from build123d import *

# Parameters (mm, degrees)
F1_DEPTH = 6.35
F3_DEPTH = 19.05
F4_SIZE  = 1.27


with BuildPart() as f1:
    # F0 (on Top) → F1 (new body)
    with BuildSketch(Plane.XY):
        with BuildLine():
            Line((-31.75, -19.05), (31.75, -19.05))
            Line((31.75, -19.05), (31.75, 12.7))
            ThreePointArc((31.75, 12.7), (29.8901280605, 17.1901280605), (25.4, 19.05))
            Line((25.4, 19.05), (12.7, 19.05))
            ThreePointArc((12.7, 19.05), (0, 6.35), (-12.7, 19.05))
            Line((-12.7, 19.05), (-25.4, 19.05))
            ThreePointArc((-25.4, 19.05), (-29.8901280605, 17.1901280605), (-31.75, 12.7))
            Line((-31.75, 12.7), (-31.75, -19.05))
        make_face()
    extrude(amount=F1_DEPTH)

    # F2 (on face) → F3 (join)
    with BuildSketch(Plane.XY.offset(6.35)):
        with BuildLine():
            Line((-25.4, 0), (-25.4, -19.05))
            Line((-25.4, -19.05), (-19.05, -19.05))
            Line((-19.05, -19.05), (-19.05, -6.35))
            Line((-19.05, -6.35), (19.05, -6.35))
            Line((19.05, -6.35), (19.05, -19.05))
            Line((19.05, -19.05), (25.4, -19.05))
            Line((25.4, -19.05), (25.4, 0))
            Line((25.4, 0), (21.59, 0))
            ThreePointArc((21.59, 0), (17.0998719395, 1.8598719395), (15.24, 6.35))
            Line((15.24, 6.35), (15.24, 19.05))
            Line((15.24, 19.05), (12.7, 19.05))
            ThreePointArc((12.7, 19.05), (0, 6.35), (-12.7, 19.05))
            Line((-12.7, 19.05), (-15.24, 19.05))
            Line((-15.24, 19.05), (-15.24, 6.35))
            ThreePointArc((-15.24, 6.35), (-17.0998719395, 1.8598719395), (-21.59, 0))
            Line((-21.59, 0), (-25.4, 0))
        make_face()
    extrude(amount=F3_DEPTH)

    # F4
    f4_edges = [f1.edges().sort_by_distance(p)[0] for p in [
        (0, 6.35, 25.4),
        (0, -6.35, 25.4),
        (-19.05, -12.7, 25.4),
        (19.05, -12.7, 25.4),
    ]]
    chamfer(f4_edges, length=F4_SIZE)


solid = f1.part
Part model, mm, in its own coordinate system. A direction names the side the tool comes from. Give positions to 0.01 mm unless a question says otherwise; leave off trailing zeros. Loops run counter-clockwise (first coordinate to the right, second up) from the corner with the lowest first, then second, coordinate; pieces in that order, holes last. Notation, with made-up numbers: M 41.5,26.5 L 61.5,26.5 A27 ccw 61.5,65.5 Z; hole C -3,39 d5. An arc over 180 degrees is marked long. Put each result on its own line as item: value. Start each with the question number.
1) 3-axis set-ups, long thin cutter, end or side, ignore diameter. For faces 1 (the flat face through (-25.4, -9, 16)), 2 (the flat face through (25.4, -10, 16)), 3 (the flat face through (15.24, 13, 16)): which of +Z, -Z, +X, -X, +Y, -Y reach the whole face in a straight line?
2) Pull direction X, two halves, no side cores. Call faces 4 (the flat face through (31.75, -3, 3)), 5 (the flat face through (24, 0, 16)), 6 (the flat face through (19.05, -13, 15)): +X half, -X half, draft (parallel to the pull), parting line (faces both ways), or undercut.
3) Saw through at A-A (x = 0). List the corners of the cut face in (y, z).
4) Saw through at B-B (y = -9). List the corners of the cut face in (x, z), then the cut area to 3 significant figures.
5) Probe probe 1 along X at (y, z) = (-8.5, 23.5); probe 2 along Z at (x, y) = (25.5, -10); probe 3 along Y at (x, z) = (-14.5, 13). List the from-to ranges inside material, lowest first.
6) Saw through at C-C (z = 13.5). List the corners of the cut face in (x, y), then the cut area to 3 significant figures.
7) Flat gauge pins, fed straight in: pin 1 (10 mm diameter, centred on y = 12, z = 11.5, fed in from +X); pin 2 (14 mm diameter, centred on x = 0, z = 18.5, fed in from -Y); pin 3 (1.5 mm diameter, centred on y = 13, z = 9.5, fed in from -X). Where does each tip first touch, or does it go through?
Numbers:
1. face 1: +Z, -X, +Y, -Y
1. face 2: +Z, +X, +Y, -Y
1. face 3: +Z, +X, +Y
2. face 4: +X half
2. face 5: draft
2. face 6: undercut
3. outline: M -19.05,0 L 6.35,0 L 6.35,24.13 L 5.08,25.4 L -5.08,25.4 L -6.35,24.13 L -6.35,6.35 L -19.05,6.35 Z
4. outline: M -31.75,0 L 31.75,0 L 31.75,6.35 L 25.4,6.35 L 25.4,25.4 L 20.32,25.4 L 19.05,24.13 L 19.05,6.35 L -19.05,6.35 L -19.05,24.13 L -20.32,25.4 L -25.4,25.4 L -25.4,6.35 L -31.75,6.35 Z
4. area: 644 mm^2
5. probe 1: -25.4 to -19.05, 19.05 to 25.4
5. probe 2: 0 to 6.35
5. probe 3: -6.35 to 19.05
6. outline: M -25.4,-19.05 L -19.05,-19.05 L -19.05,-6.35 L 19.05,-6.35 L 19.05,-19.05 L 25.4,-19.05 L 25.4,0 L 21.59,0 A6.35 cw 15.24,6.35 L 15.24,19.05 L 12.7,19.05 A12.7 cw -12.7,19.05 L -15.24,19.05 L -15.24,6.35 A6.35 cw -21.59,0 L -25.4,0 Z
6. area: 828 mm^2
7. pin 1: x = 15.24
7. pin 2: y = -6.35
7. pin 3: x = -15.24
